```python
from build123d import *

# Parameters (mm, degrees)
F7_DEPTH      = 8.9543153527
F7_DEPTH_BACK = 25.4


with BuildPart() as f1:
    # F0 (on Right) → F1 (revolve)
    with BuildSketch(Plane.YZ):
        Polygon((-38.496875, 0), (0, 0), (0, 6.33095), (-36.5125, 6.33095), (-36.5125, 4.9784), (-38.496875, 4.9784), align=None)
    revolve(axis=Axis((0, 7.9408854224, 0), (0, 1, 0)))

    # F2 (on Right) → F3 (revolve, cut)
    with BuildSketch(Plane.YZ):
        Polygon((0, 5.6896), (-34.13125, 5.6896), (-35.6557737253, 0), (0, 0), align=None)
    revolve(axis=Axis((0, 5.2174264412, 0), (0, 1, 0)), mode=Mode.SUBTRACT)

    # F6 (on line) → F7 (cut, two sides)
    with BuildSketch(Plane(origin=(0, 0, 0), x_dir=(0, -1, 0), z_dir=(-0.7071067812, 0, -0.7071067812))) as f7_sk:
        Polygon((37.506275, 4.9784), (38.496875, 4.4831), (37.506275, 3.9878), (38.496875, 3.4925), (37.506275, 2.9972), (38.496875, 2.5019), (37.506275, 2.0066), (38.496875, 1.5113), (37.506275, 1.016), (38.496875, 0.5207), (38.496875, -0.5207), (37.506275, -1.016), (38.496875, -1.5113), (37.506275, -2.0066), (38.496875, -2.5019), (37.506275, -2.9972), (38.496875, -3.4925), (37.506275, -3.9878), (38.496875, -4.4831), (37.506275, -4.9784), (37.506275, -6.6715925932), (39.5995303988, -6.6715925932), (39.5995303988, 6.7129228264), (37.506275, 6.7129228264), align=None)
    extrude(amount=-F7_DEPTH, mode=Mode.SUBTRACT)
    extrude(f7_sk.sketch, amount=F7_DEPTH_BACK, mode=Mode.SUBTRACT)


solid = f1.part
```
For this review, take the finished solid that the model builds, in its own axes (mm). A direction names the side the tool comes from. Round coordinates to 2 decimals unless told otherwise and drop trailing zeros. Write each loop counter-clockwise with the first axis right and the second up, starting at its lowest first coordinate (ties: lowest second). Pieces come first, ordered by that corner, then holes. Notation, with made-up numbers: M 35.25,48 L 46.25,48 A30 ccw 46.25,86 Z; hole C 78.25,64 d4. An arc over 180 degrees is marked long. One line per item, written item: value. Start each with the question number.
(1) Machinability: for faces 1 (the cylindrical face through (-5.554, -17.305, -1.233)), 2 (the cylindrical face through (-4.417, -37.298, 2.297)), 3 (the cylindrical face through (0.278, -18.512, -6.325)), which of the approach directions +Z, -Z, +X, -X, +Y, -Y give a long, thin tool a straight path to every point of the face, cutting with its end or side? Answer none if there is none.
(2) We need section A-A (y = -24.5). Give the boundary of the cut face in (x, z).
(3) Wall thickness on line 1 (X direction, y = -9, z = 0); line 2 (Z direction, x = 1.5, y = -15.5); line 3 (Z direction, x = -2.75, y = -17.5): over which ranges is each line inside the solid? List them lowest first.
(4) Insertion check: pin 1 (6 mm diameter, centred on x = 1, z = -2, fed in from +Y); pin 2 (6 mm diameter, centred on y = -14.5, z = -1, fed in from -X); pin 3 (3 mm diameter, centred on y = -22, z = -4, fed in from -X); pin 4 (2 mm diameter, centred on x = -2.5, y = -16, fed in from -Z). Each pin has a flat end and moves straight along its axis. Give the tip position at first contact, or say it passes through.
Result:
1. face 1: +Y
1. face 2: -Y
1. face 3: +Y, -Y
2. outline: C 0,0 d12.66; hole C 0,0 d11.38
3. line 1: -6.33 to -5.69, 5.69 to 6.33
3. line 2: -6.15 to -5.49, 5.49 to 6.15
3. line 3: -5.7 to -4.98, 4.98 to 5.7
4. pin 1: y = -34.25
4. pin 2: x = -6.33
4. pin 3: x = -5.82
4. pin 4: z = -6.15
